from build123d import *

# Parameters (mm, degrees)
F1_DEPTH = 3.5
F2_R     = 5
F3_R     = 0.8
F4_R     = 3
F5_R     = 0.5


with BuildPart() as f1:
    # F0 (on Top) → F1 (new body)
    with BuildSketch(Plane.XY):
        with BuildLine():
            Line((27.0056332441, 1.6), (4.3127717306, 1.6))
            ThreePointArc((4.3127717306, 1.6), (-4.1689707148, 1.9441407303), (1.5463240937, -4.3323067525))
            Line((1.5463240937, -4.3323067525), (-0.0881351041, -1.9980571072))
            ThreePointArc((-0.0881351041, -1.9980571072), (-1.0206418303, 1.7199680969), (1.7959955457, -0.88))
            ThreePointArc((1.7959955457, -0.88), (1.8207303634, -1.3645751311), (2.2449944321, -1.6))
            Line((2.2449944321, -1.6), (4.3127717306, -1.6))
            Line((4.3127717306, -1.6), (27.8630706599, -1.6))
            ThreePointArc((27.8630706599, -1.6), (33.039451562, -0.9185165258), (37.8630706599, 1.0794919243))
            Line((37.8630706599, 1.0794919243), (41.5192378865, 3.1903810568))
            ThreePointArc((41.5192378865, 3.1903810568), (45.1369522099, 4.6888873943), (49.0192378865, 5.2))
            Line((49.0192378865, 5.2), (51, 5.2))
            Line((51, 5.2), (51, 8.4))
            Line((51, 8.4), (48.1618004707, 8.4))
            ThreePointArc((48.1618004707, 8.4), (44.2795147941, 7.8888873943), (40.6618004707, 6.3903810568))
            Line((40.6618004707, 6.3903810568), (37.0056332441, 4.2794919243))
            ThreePointArc((37.0056332441, 4.2794919243), (32.1820141462, 2.2814834742), (27.0056332441, 1.6))
        make_face()
    extrude(amount=F1_DEPTH)

    # F2
    f2_edges = [f1.edges().sort_by_distance(p)[0] for p in [
        (4.312772, 1.6, 1.75),
        (27.863071, -1.6, 1.75),
    ]]
    fillet(f2_edges, radius=F2_R)

    # F3
    f3_edges = [f1.edges().sort_by_distance(p)[0] for p in [
        (1.546324, -4.332307, 1.75),
    ]]
    fillet(f3_edges, radius=F3_R)

    # F4
    f4_edges = [f1.edges().sort_by_distance(p)[0] for p in [
        (51, 8.4, 1.75),
    ]]
    fillet(f4_edges, radius=F4_R)

    # F5
    f5_edges = [f1.edges().sort_by_distance(p)[0] for p in [
        (51, 5.2, 1.75),
    ]]
    fillet(f5_edges, radius=F5_R)


solid = f1.part
Here's how the part is built. I have some questions about the finished solid (model axes, mm). A direction names the side the tool comes from. Coordinates: 2 decimals unless noted, no trailing zeros. Order: outer loops, then holes, each group sorted by start corner. A loop starts at its lowest first (then second) coordinate and runs counter-clockwise, first axis right, second up.
Item 1: For P1, Ø1.5, axis at y = -2.5, z = 2, coming from the +X side; P2, Ø2, axis at x = 19, z = 2.5, coming from the -Y side; P3, Ø2, axis at x = 43.5, z = 1.5, coming from the -Y side, each with a flat end and sliding along its axis, tell me the tip position at first contact or that it passes through.
Result sheet:
P1: stops at x = 0.79
P2: stops at y = -1.6
P3: stops at y = 3.71
Item 2: I need wall thicknesses on line 1 (Y direction, x = 17, z = 0.25); line 2 (Y direction, x = 0, z = 1.65); line 3 (X direction, y = 0, z = 2.45). Which ranges of each line are inside material? Lowest first, please.
Result sheet:
line 1: y = -1.6 to 1.6
line 2: y = -4.6 to -2.12, 2 to 4.6
line 3: x = -4.6 to -2, 2 to 35.7
Item 3: If we mould it in two halves opening along X, with no side actions, what happens to faces 1 (the face through (32.969, -0.937, 1.726)), 2 (the face through (21, 1, 0)), 3 (the face through (-1.082, 1.682, 1.726))? For each: +X half, -X half, draft (parallel to the pull), parting line (faces both ways), or undercut.
Result sheet:
face 1: +X half
face 2: draft
face 3: undercut
Item 4: For faces 4 (the face through (0.39, -2.68, 1.73)), 5 (the face through (21, 1, 3.5)), 6 (the face through (17, 1.6, 2)), 7 (the face through (44.234, 7.877, 1.726)), 8 (the face through (50, 5.2, 2)), which set-ups out of +Z, -Z, +X, -X, +Y, -Y let a thin tool reach every point of the face, with its end or its side?
Result sheet:
face 4: +Z, -Z, +X
face 5: +Z, +X, -X, +Y, -Y
face 6: +Z, -Z, +Y
face 7: +Z, -Z, -X, +Y
face 8: +Z, -Z, +X, -Y
Item 5: If we section it at A-A on y = 0: List the corners of the cut face in (x, z) for me, plus the area to 3 significant figures.
Result sheet:
outline: (-4.6, 0) - (-2, 0) - (-2, 3.5) - (-4.6, 3.5) - close; (2, 0) - (35.7, 0) - (35.7, 3.5) - (2, 3.5) - close
area: 127 mm2
Item 6: If we section it at B-B on x = 23.5: List the corners of the cut face in (y, z) for me, plus the area to 3 significant figures.
Result sheet:
outline: (-1.6, 0) - (1.6, 0) - (1.6, 3.5) - (-1.6, 3.5) - close
area: 11.2 mm2
